from build123d import *
from build123d.topology import SkipClean

# Parameters (mm, degrees)
CUT_EXTRUDE4_START = 15
CUT_EXTRUDE4_DEPTH = 80
CUT_EXTRUDE6_START = -65
SKETCH6_R          = 12.5
CUT_EXTRUDE6_DEPTH = 80


with BuildPart() as part:
    # Sketch1 → Revolve1 (revolve)
    with BuildSketch(Plane.XY):
        with BuildLine():
            Line((46.097722286, -30), (0, -30))
            Line((0, -30), (0, 55))
            ThreePointArc((0, 55), (48.347699015, 26.220221204), (46.097722286, -30))
        make_face()
    revolve(axis=Axis((0, 4.730452026, 0), (0, 1, 0)))

    # Sketch3 → Cut-Extrude4 (cut)
    with BuildSketch(Plane(origin=(0, 0, 0), x_dir=(1, 0, 0), z_dir=(0, 1, 0)).offset(CUT_EXTRUDE4_START)):
        with BuildLine():
            Line((-25, 12.5), (25, 12.5))
            ThreePointArc((25, 12.5), (37.5, 0), (25, -12.5))
            Line((25, -12.5), (-25, -12.5))
            ThreePointArc((-25, -12.5), (-37.5, 0), (-25, 12.5))
        make_face()
    extrude(amount=CUT_EXTRUDE4_DEPTH, mode=Mode.SUBTRACT)

    # Sketch6 → Cut-Extrude6 (cut)
    with SkipClean():  # the faces are left unmerged after this step: merging them gives an invalid solid
        with BuildSketch(Plane(origin=(0, 0, 0), x_dir=(1, 0, 0), z_dir=(0, 1, 0)).offset(CUT_EXTRUDE6_START)):
            with Locations(Location((-25, 0, 0), (0, 0, 90))):
                Circle(SKETCH6_R)
            with Locations(Location((25, 0, 0), (0, 0, 90))):
                Circle(SKETCH6_R)
        extrude(amount=CUT_EXTRUDE6_DEPTH, mode=Mode.SUBTRACT)


solid = part.part
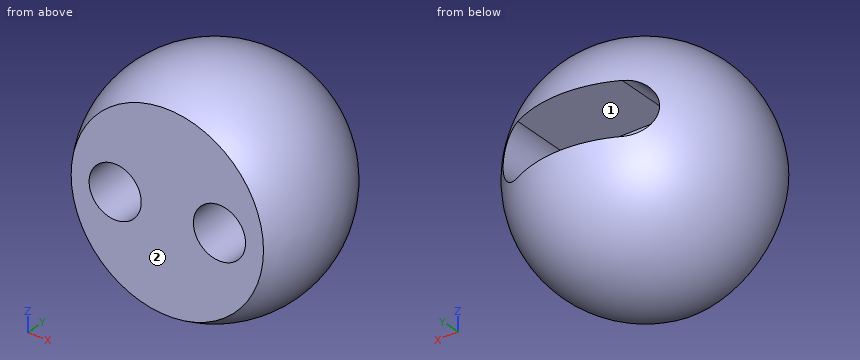
The model under review builds one solid part; all positions refer to its coordinate system, in mm. Face numbers are marked on the shaded views. Round coordinates to 2 decimals unless told otherwise and drop trailing zeros. Loops run counter-clockwise (first coordinate to the right, second up) from the corner with the lowest first, then second, coordinate; pieces in that order, holes last. Notation, with made-up numbers: (-36, 46) -> (-13, 46) arc R19 ccw to (-13, 50) -> close; hole circle Ø2 at (5.25, 68.25). An arc over 180 degrees is marked (long way). Write item = value, one per line. Start each with the question number.
Item 1: Mouldability with a two-part tool opening along Z and no side actions: class the marked faces 1 and 2 as released by +Z, released by -Z, zero draft, split by the parting line, or undercut.
Item 2: Insertion check: pin 1 (1.5 mm diameter, centred on x = -23, y = 5.5, fed in from +Z); pin 2 (20 mm diameter, centred on x = 10.5, z = 2, fed in from +Y); pin 3 (3 mm diameter, centred on y = 31.5, z = -38.5, fed in from -X). Each pin has a flat end and moves straight along its axis. Give the tip position at first contact, or say it passes through.
Item 3: Take a section at B-B on x = -16. Give the boundary of the cut face in (y, z), plus the area to 3 significant figures.
Item 4: Take a section at A-A on z = 0. Give the boundary of the cut face in (x, y).
Item 5: Take a section at D-D on z = 28. Give the boundary of the cut face in (x, y).
Item 6: To check wall thickness, follow L1, parallel to X at y = 2, z = 0; L2, parallel to X at y = -8, z = 0; L3, parallel to Z at x = -25, y = 5.5. State the ranges of each line that lie inside material, in increasing order.
Item 7: Take a section at C-C on y = -2.5. Give the boundary of the cut face in (x, z), plus the area to 3 significant figures.
Result:
q1.face_1 = undercut
q1.face_2 = zero draft
q2.pin_1 = 50.01
q2.pin_2 = 15
q2.pin_3 = -26.41
q3.outline = (-30, -43.23) arc R52.62 ccw to (51.12, -12.5) -> (15, -12.5) -> (15, -8.67) -> (-30, -8.67) -> close; (-30, 8.67) -> (15, 8.67) -> (15, 12.5) -> (51.12, 12.5) arc R52.62 ccw to (-30, 43.23) -> close
q3.area = 5,620 mm²
q4.outline = (-46.1, -30) -> (-37.5, -30) -> (-37.5, 40.23) arc R55 ccw to start; (-12.5, -30) -> (12.5, -30) -> (12.5, 15) -> (-12.5, 15) -> close; (37.5, -30) -> (46.1, -30) arc R55 ccw to (37.5, 40.23) -> close
q5.outline = (-36.62, -30) -> (36.62, -30) arc R47.34 ccw (long way) to start
q6.L1 = -54.96 to -37.5, -12.5 to 12.5, 37.5 to 54.96
q6.L2 = -54.42 to -37.5, -12.5 to 12.5, 37.5 to 54.42
q6.L3 = -48.68 to -12.5, 12.5 to 48.68
q7.outline = circle Ø109.89 at (0, 0); hole circle Ø25 at (-25, 0); hole circle Ø25 at (25, 0)
q7.area = 8,500 mm²
